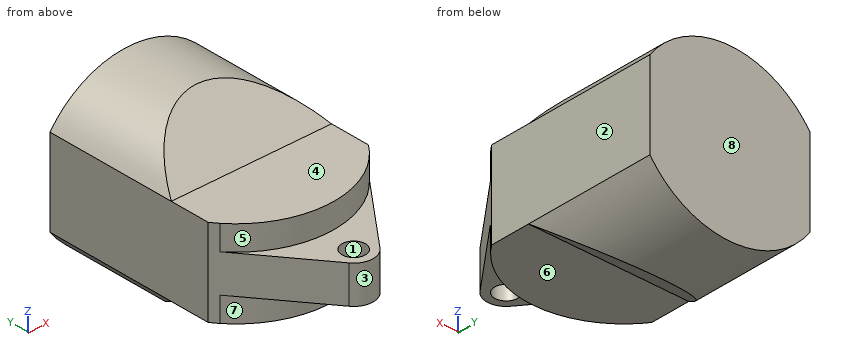
from build123d import *

# Parameters (mm, degrees)
EXTRUDE_1_DEPTH     = 67
SKETCH_2_OUTSIDE_W  = 175.426
SKETCH_2_OUTSIDE_H  = 254.426
CUT_EXTRUDE_1_DEPTH = 19
SKETCH_4_OUTSIDE_W  = 175.426
SKETCH_4_OUTSIDE_H  = 254.426
CUT_EXTRUDE_2_DEPTH = 19
EXTRUDE_2_DEPTH     = 102
CUT_EXTRUDE_3_DEPTH = 247.010162392
SKETCH_7_R          = 9
CUT_EXTRUDE_4_DEPTH = 214.513465618


with BuildPart() as part:
    # Эскиз1 → Бобышка-Вытянуть1 (new body)
    with BuildSketch(Plane.XY):
        with BuildLine():
            Line((-62, 55), (-62, 188))
            Line((-62, 188), (62, 188))
            Line((62, 188), (62, 55))
            Line((62, 55), (12.047963129, -8.935691604))
            ThreePointArc((12.047963129, -8.935691604), (0, -15), (-12.047963129, -8.935691604))
            Line((-12.047963129, -8.935691604), (-62, 55))
        make_face()
    extrude(amount=EXTRUDE_1_DEPTH)

    # Эскиз2 outside → Вырез-Вытянуть1 (cut)
    with BuildSketch(Plane.XY.offset(67)):
        with Locations((0, 86.5)):
            Rectangle(SKETCH_2_OUTSIDE_W, SKETCH_2_OUTSIDE_H)
        with BuildLine():
            Line((-62, 55), (-62, 188))
            Line((-62, 188), (62, 188))
            Line((62, 188), (62, 55))
            ThreePointArc((62, 55), (0, 23), (-62, 55))
        make_face(mode=Mode.SUBTRACT)
    extrude(amount=-CUT_EXTRUDE_1_DEPTH, mode=Mode.SUBTRACT)

    # Эскиз4 outside → Вырез-Вытянуть2 (cut)
    with BuildSketch(Plane(origin=(0, 0, 0), x_dir=(-1, 0, 0), z_dir=(0, 0, -1))):
        with Locations((0, 86.5)):
            Rectangle(SKETCH_4_OUTSIDE_W, SKETCH_4_OUTSIDE_H)
        with BuildLine():
            Line((-62, 55), (-62, 188))
            Line((-62, 188), (62, 188))
            Line((62, 188), (62, 55))
            ThreePointArc((62, 55), (0, 23), (-62, 55))
        make_face(mode=Mode.SUBTRACT)
    extrude(amount=-CUT_EXTRUDE_2_DEPTH, mode=Mode.SUBTRACT)

    # Эскиз5 → Бобышка-Вытянуть2 (add)
    with BuildSketch(Plane(origin=(0, 188, 0), x_dir=(1, 0, 0), z_dir=(0, 1, 0))):
        with BuildLine():
            Line((-62, 0), (62, 0))
            ThreePointArc((62, 0), (0, 32), (-62, 0))
        make_face()
        with BuildLine():
            Line((-62, -67), (62, -67))
            ThreePointArc((62, -67), (0, -99), (-62, -67))
        make_face()
    extrude(amount=-EXTRUDE_2_DEPTH)

    # Эскиз6 → Вырез-Вытянуть3 (cut, through all)
    with BuildSketch(Plane(origin=(62, 0, 0), x_dir=(0, 0, -1), z_dir=(1, 0, 0))):
        Polygon((0, 86), (32, 131.700736216), (32, 86), align=None)
        Polygon((-67, 86), (-99, 131.700736216), (-99, 86), align=None)
    extrude(amount=-CUT_EXTRUDE_3_DEPTH, mode=Mode.SUBTRACT)

    # Эскиз7 → Вырез-Вытянуть4 (cut, through all)
    with BuildSketch(Plane(origin=(0, 0, 19), x_dir=(-1, 0, 0), z_dir=(0, 0, -1))):
        Circle(SKETCH_7_R)
    extrude(amount=-CUT_EXTRUDE_4_DEPTH, mode=Mode.SUBTRACT)


solid = part.part
Work out the finished part from the listing and answer in its coordinate system (mm). Face numbers are marked on the shaded views. A direction names the side the tool comes from. Coordinates: 2 decimals unless noted, no trailing zeros. Write each loop counter-clockwise with the first axis right and the second up, starting at its lowest first coordinate (ties: lowest second). Pieces come first, ordered by that corner, then holes.
1. The part is cut by section C-C, the plane y = 0. Write down the section's boundary in (x, z).
Results list:
outline: (-19.03, 19) - (-9, 19) - (-9, 48) - (-19.03, 48) - close; (9, 19) - (19.03, 19) - (19.03, 48) - (9, 48) - close
2. The part is cut by section D-D, the plane z = 60. Write down the section's boundary in (x, y) (1 decimal).
Results list:
outline: (-62, 55) - (-57.8, 49.6) arc R76.1 ccw to (57.8, 49.6) - (62, 55) - (62, 188) - (-62, 188) - close
3. For the marked faces 4, 5, 6, 7 and 8, determine the directions among +Z, -Z, +X, -X, +Y, -Y from which every point of the face is accessible in a straight line to the end or side of a thin tool.
Results list:
face 4: +Z, +X, -X, -Y
face 5: +Z, -Y
face 6: -Z, +X, -X, -Y
face 7: -Z, -Y
face 8: +Z, -Z, +X, -X, +Y
4. The part is cut by section B-B, the plane z = 45.5. Write down the section's boundary in (x, y).
Results list:
outline: (-62, 55) - (-12.05, -8.94) arc R15 ccw to (12.05, -8.94) - (62, 55) - (62, 188) - (-62, 188) - close; hole circle Ø18 at (0, 0)
5. Flat-ended cylindrical pins translate along their axes: pin 1 (1.5 mm diameter, centred on x = -47, y = 87.5, fed in from +Z); pin 2 (2 mm diameter, centred on x = 7.5, y = 26, fed in from -Z); pin 3 (5 mm diameter, centred on y = 46.5, z = 18.5, fed in from +X). Find the tip coordinate at first contact, or state that the pin passes through.
Results list:
pin 1: stops at z = 68.58
pin 2: stops at z = 0
pin 3: stops at x = 57.27
6. The part is cut by section A-A, the plane x = 0. Write down the section's boundary in (y, z), and give its area (3 significant figures).
Results list:
outline: (-15, 19) - (-9, 19) - (-9, 48) - (-15, 48) - close; (9, 19) - (23, 19) - (23, 0) - (86, 0) - (131.7, -32) - (188, -32) - (188, 99) - (131.7, 99) - (86, 67) - (23, 67) - (23, 48) - (9, 48) - close
area: 16,700 mm2
7. Consider line 1 along Y through (x, z) = (0, 25); line 2 along Z through (x, y) = (17, 21); line 3 along Y through (x, z) = (-19, 46.5). Determine where each line is inside the solid, lowest interval first.
Results list:
line 1: y = -15 to -9, 9 to 188
line 2: z = 19 to 48
line 3: y = -0.04 to 188
8. For a pull along Y with two mould halves and no side action, classify the marked faces 1, 2 and 3 as +Y half, -Y half, draft (parallel to the pull), parting line (faces both ways), or undercut.
Results list:
face 1: undercut
face 2: draft
face 3: -Y half
